from build123d import *

# Parameters (mm, degrees)
ESQUISSE1_W             = 5
ESQUISSE1_H             = 20
BOSS_EXTRU_1_DEPTH      = 20.5
ESQUISSE2_W             = 25
ESQUISSE2_H             = 20
BOSS_EXTRU_2_DEPTH      = 2
ESQUISSE3_R             = 3.175
BOSS_EXTRU_3_DEPTH      = 7
CONG_1_R                = 10
ESQUISSE4_R             = 1.05
ENL_V_MAT_EXTRU_1_DEPTH = 8


with BuildPart() as part:
    # Esquisse1 → Boss.-Extru.1 (new body)
    with BuildSketch(Plane.XY):
        Rectangle(ESQUISSE1_W, ESQUISSE1_H)
    extrude(amount=BOSS_EXTRU_1_DEPTH)

    # Esquisse2 → Boss.-Extru.2 (add)
    with BuildSketch(Plane.XY.offset(20.5)):
        with Locations((-10, 0)):
            Rectangle(ESQUISSE2_W, ESQUISSE2_H)
    extrude(amount=BOSS_EXTRU_2_DEPTH)

    # Esquisse3 → Boss.-Extru.3 (add)
    with BuildSketch(Plane.XY.offset(22.5)):
        with Locations((-12.41, 0.35)):
            Circle(ESQUISSE3_R)
    extrude(amount=BOSS_EXTRU_3_DEPTH)

    # Congé1
    cong_1_edges = [part.edges().sort_by_distance(p)[0] for p in [
        (-22.5, 10, 21.5),
        (-22.5, -10, 21.5),
    ]]
    fillet(cong_1_edges, radius=CONG_1_R - 0.0001)  # a hair under: the kernel refuses the full size

    # Esquisse4 → Enlèv. mat.-Extru.1 (cut)
    with BuildSketch(Plane(origin=(0, 0, 0), x_dir=(-1, 0, 0), z_dir=(0, 0, -1))):
        with Locations((0, 5)):
            Circle(ESQUISSE4_R)
        with Locations((0, -5)):
            Circle(ESQUISSE4_R)
    extrude(amount=-ENL_V_MAT_EXTRU_1_DEPTH, mode=Mode.SUBTRACT)


solid = part.part
CAD build for the part. Positions are in the model's coordinates, mm. A direction names the side the tool comes from. Coordinates: 2 decimals unless noted, no trailing zeros. Write each loop counter-clockwise with the first axis right and the second up, starting at its lowest first coordinate (ties: lowest second). Pieces come first, ordered by that corner, then holes. Notation, with made-up numbers: M -30.75,-31.5 L 9.25,-31.5 A6 cw 9.25,-20.5 Z; hole C -35.75,68.25 d1. An arc over 180 degrees is marked long. Return JSON: item names as keys, results as strings.
Item 1: Which spindle directions (+Z, -Z, +X, -X, +Y, -Y) get a long thin tool onto all of the face, cutting with end or side? Do faces 4 (the flat face through (-13, 0, 20.5)), 5 (the cylindrical face through (0.14, 6.04, 3.94)), 6 (the cylindrical face through (-9.38, 1.3, 25.95)). Say none if no direction does.
Findings below:
{"face 4": "-Z, -X, +Y, -Y", "face 5": "-Z", "face 6": "+Z"}
Item 2: Two-plate mould, pull along X, no slides. Class faces 1 (the flat face through (0, 5, 8)), 2 (the cylindrical face through (-19.65, -6.99, 21.51)), 3 (the flat face through (0, 0, 0)): +X half, -X half, draft (parallel to the pull), parting line (faces both ways), or undercut.
Findings below:
{"face 1": "undercut", "face 2": "-X half", "face 3": "draft"}
Item 3: Drop flat-ended pins along their axis: pin 1 Ø2 at (x, y) = (-14, -8) entering from -Z; pin 2 Ø1.9 at (x, y) = (0, -5) entering from +Z; pin 3 Ø1.9 at (x, y) = (0, 5) entering from -Z. Give the stop position or say it passes through.
Findings below:
{"pin 1": "stops at z = 20.5", "pin 2": "stops at z = 22.5", "pin 3": "stops at z = 8"}
Item 4: Probe line 1 (Y direction, x = 0, z = 6.5); line 2 (Z direction, x = -3.75, y = -1); line 3 (Z direction, x = 0, y = -8.75). List the from-to ranges inside material, lowest first. Write a range as from..to.
Findings below:
{"line 1": "y = -10..-6.05, -3.95..3.95, 6.05..10", "line 2": "z = 20.5..22.5", "line 3": "z = 0..22.5"}
Item 5: Slice it at C-C, the plane y = 1.25. Write the cut outline in (x, z).
Findings below:
{"outline": "M -22.42,20.5 L -2.5,20.5 L -2.5,0 L 2.5,0 L 2.5,22.5 L -9.37,22.5 L -9.37,29.5 L -15.45,29.5 L -15.45,22.5 L -22.42,22.5 Z"}
Item 6: Slice it at D-D, the plane y = -5. Write the cut outline in (x, z), and give its area (3 significant figures).
Findings below:
{"outline": "M -21.16,20.5 L -2.5,20.5 L -2.5,0 L -1.05,0 L -1.05,8 L 1.05,8 L 1.05,0 L 2.5,0 L 2.5,22.5 L -21.16,22.5 Z", "area": "133 mm2"}
Item 7: Slice it at B-B, the plane z = 26. Write the cut outline in (x, y) (3 decimals).
Findings below:
{"outline": "C -12.41,0.35 d6.35"}
Item 8: Slice it at A-A, the plane x = 0. Write the cut outline in (y, z), and give its area (3 significant figures).
Findings below:
{"outline": "M -10,0 L -6.05,0 L -6.05,8 L -3.95,8 L -3.95,0 L 3.95,0 L 3.95,8 L 6.05,8 L 6.05,0 L 10,0 L 10,22.5 L -10,22.5 Z", "area": "416 mm2"}
